Could you check a few things on this model? Use its own coordinates, in mm. Face numbers are marked on the shaded views. Coordinates: 2 decimals unless noted, no trailing zeros. Loops run counter-clockwise (first coordinate to the right, second up) from the corner with the lowest first, then second, coordinate; pieces in that order, holes last. Notation, with made-up numbers: (40, -10) - (69, -10) arc R12 cw to (69, 13) - close; hole circle Ø6 at (39.25, 13). An arc over 180 degrees is marked (long way). One line per item, written item: value. Start each with the question number.
(1) If I drill on line 1 along X through (y, z) = (1.85, -1.5); line 2 along X through (y, z) = (0.35, -0.5); line 3 along Z through (x, y) = (-0.75, 0.15), over which ranges is the centre line in solid material (lowest first)? Write a range as from..to.
(2) If we mould it in two halves opening along X, with no side actions, what happens to the marked faces 1, 2, 3 and 4? For each: pulls with the +X half, pulls with the -X half, needs draft (parallel to the pull), parting line crosses it, or undercut.
(3) If we section it at A-A on y = 2.3: Write out the boundary of the cut face in (x, z), then the cut area to 3 significant figures.
(4) I'm going to push a flat-ended pin straight in: P1, Ø1.5, axis at y = 2, z = -1.5, coming from the +X side. Where does the tip first touch, or does it pass through?
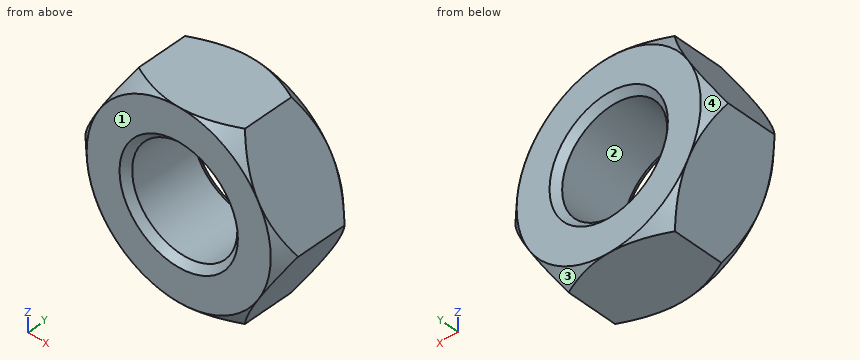
```python
from build123d import *

# Parameters (mm, degrees)
SKETCH1_R           = 2
BOSS_EXTRUDE1_DEPTH = 3
CHAMFER2_SIZE       = 0.25


with BuildPart() as part:
    # Sketch1 → Boss-Extrude1 (new body)
    with BuildSketch(Plane(origin=(0, 0, 0), x_dir=(1, 0, 0), z_dir=(0, 1, 0))):
        Polygon((-2.020725942, -3.5), (2.020725942, -3.5), (4.041451884, 0), (2.020725942, 3.5), (-2.020725942, 3.5), (-4.041451884, 0), align=None)
        Circle(SKETCH1_R, mode=Mode.SUBTRACT)
    extrude(amount=BOSS_EXTRUDE1_DEPTH)

    # Sketch2 → Cut-Revolve1 (revolve, cut)
    with BuildSketch(Plane(origin=(0, 0, 0), x_dir=(0, 0, -1), z_dir=(1, 0, 0))):
        Polygon((3.5, 3), (4.55, 4.05), (4.55, 1.95), align=None)
        Polygon((4.55, 1.05), (3.5, 0), (4.55, -1.05), align=None)
    revolve(axis=Axis((0, 3, 0), (0, -1, 0)), mode=Mode.SUBTRACT)

    # Chamfer2
    chamfer2_edges = [part.edges().sort_by_distance(p)[0] for p in [
        (-2, 0, 0),
        (-2, 3, 0),
    ]]
    chamfer(chamfer2_edges, length=CHAMFER2_SIZE)


solid = part.part
```
Values:
1. line 1: x = -3.18..-1.32, 1.32..3.18
1. line 2: x = -3.75..-1.94, 1.94..3.75
1. line 3: z = -3.5..-1.96, 1.96..3.5
2. face 1: needs draft
2. face 2: undercut
2. face 3: pulls with the +X half
2. face 4: pulls with the -X half
3. outline: (-4.04, 0) - (-2.02, -3.5) - (2.02, -3.5) - (4.04, 0) - (2.02, 3.5) - (-2.02, 3.5) - close; hole circle Ø4 at (0, 0)
3. area: 29.9 mm2
4. P1: stops at x = 3.61
